For this review, take the finished solid that the model builds, in its own axes (mm). A direction names the side the tool comes from. Coordinates: 2 decimals unless noted, no trailing zeros. Loops run counter-clockwise (first coordinate to the right, second up) from the corner with the lowest first, then second, coordinate; pieces in that order, holes last. Notation, with made-up numbers: (60.25, -13) - (67.25, -13) arc R18 ccw to (67.25, 4) - close; hole circle Ø9 at (29.25, 1). An arc over 180 degrees is marked (long way). Answer as a JSON object with one key per item and string values. Group by question number.
Item 1: We need section A-A (y = 11.25). Give the boundary of the cut face in (x, z), then the cut area to 3 significant figures.
Item 2: We need section D-D (x = 21). Give the boundary of the cut face in (y, z).
Item 3: We need section C-C (y = 24.5). Give the boundary of the cut face in (x, z), then the cut area to 3 significant figures.
Item 4: Mouldability with a two-part tool opening along Y and no side actions: class faces 4 (the flat face through (56, 26.416, -18)), 5 (the cylindrical face through (57.34, 10.39, -18.41)), 6 (the cylindrical face through (4.996, 19.056, -18.406)), 7 (the flat face through (10.287, 16, -18)) as released by +Y, released by -Y, zero draft, split by the parting line, or undercut.
Item 5: Clearance check with flat-ended pins moving along their axes: pin 1 (4 mm diameter, centred on x = 55.26, y = 21.25, fed in from +Z); pin 2 (3 mm diameter, centred on x = 54.5, z = -3.5, fed in from +Y); pin 3 (1 mm diameter, centred on x = 37.5, z = -18.5, fed in from +Y); pin 4 (3 mm diameter, centred on x = 8, y = 14, fed in from +Z). State where each tip first meets the part, or that it passes through.
Item 6: To check wall thickness, follow line 1 (X direction, y = 0.9, z = -7.62); line 2 (Y direction, x = 18, z = -8.5); line 3 (X direction, y = 12.25, z = -18). State the ranges of each line that lie inside material, in increasing order.
Item 7: We need section B-B (z = -7.62). Give the boundary of the cut face in (x, y).
Item 8: Tool access review of faces 1 (the flat face through (60.96, 9, -18)), 2 (the flat face through (30, 1.27, -8)), 3 (the flat face through (30, 6.35, -18)): name each direction out of +Z, -Z, +X, -X, +Y, -Y from which nothing blocks a thin tool from reaching the whole face with its end or side.
from build123d import *

# Parameters (mm, degrees)
BOSS_EXTRUDE1_DEPTH    = 60.96
CONVERT_SOLID1_DEPTH   = 60.96
CONVERT_SOLID1_2_DEPTH = 60.96
SKETCH6_W              = 40.386
SKETCH6_H              = 20.066
CUT_EXTRUDE1_DEPTH     = 71.995158286
SKETCH8_R              = 1.89865
CUT_EXTRUDE2_DEPTH     = 71.767609116
SKETCH9_R              = 2.2479
CUT_EXTRUDE3_DEPTH     = 71.995158286
CUT_EXTRUDE4_DEPTH     = 71.995158286


# Read off the part's stored shape, not the designer's step: Convert-Solid1
with BuildPart() as part:
    # Sketch1 → Boss-Extrude1 (new body)
    with BuildSketch(Plane(origin=(0, 0, 0), x_dir=(0, 0, -1), z_dir=(1, 0, 0))):
        Polygon((0, 0), (19.05, 0), (19.05, 31.75), (17.78, 31.75), (17.78, 1.27), (0, 1.27), align=None)
    extrude(amount=BOSS_EXTRUDE1_DEPTH)

    # Convert-Solid1 outline → Convert-Solid1 (cut)
    with BuildSketch(Plane.YZ):
        with BuildLine():
            ThreePointArc((2.54, -19.05), (0.743948776, -18.306051224), (0, -16.51))
            Line((0, -16.51), (0, -19.05))
            Line((0, -19.05), (2.54, -19.05))
        make_face()
    extrude(amount=CONVERT_SOLID1_DEPTH, mode=Mode.SUBTRACT)

    # Convert-Solid1 2 outline → Convert-Solid1 2 (add)
    with BuildSketch(Plane.YZ):
        with BuildLine():
            ThreePointArc((2.54, -17.78), (1.641974388, -17.408025612), (1.27, -16.51))
            Line((1.27, -16.51), (1.27, -17.78))
            Line((1.27, -17.78), (2.54, -17.78))
        make_face()
    extrude(amount=CONVERT_SOLID1_2_DEPTH)

    # Sketch6 → Cut-Extrude1 (cut, through all)
    with BuildSketch(Plane.XY.offset(-17.78)):
        with Locations((30.48, 16.383)):
            Rectangle(SKETCH6_W, SKETCH6_H)
    extrude(amount=-CUT_EXTRUDE1_DEPTH, mode=Mode.SUBTRACT)

    # Sketch8 → Cut-Extrude2 (cut, through all)
    with BuildSketch(Plane(origin=(0, 1.27, 0), x_dir=(1, 0, 0), z_dir=(0, 1, 0))):
        with Locations(Location((7.62, 7.62, 0), (0, 0, 270))):
            Circle(SKETCH8_R)
        with Locations(Location((53.34, 7.62, 0), (0, 0, 270))):
            Circle(SKETCH8_R)
    extrude(amount=-CUT_EXTRUDE2_DEPTH, mode=Mode.SUBTRACT)

    # Sketch9 → Cut-Extrude3 (cut, through all)
    with BuildSketch(Plane.XY.offset(-17.78)):
        with Locations((5.483386699, 21.25)):
            Circle(SKETCH9_R)
        with Locations((5.483386699, 11.25)):
            Circle(SKETCH9_R)
        with Locations((55.262613301, 21.25)):
            Circle(SKETCH9_R)
        with Locations((55.262613301, 11.25)):
            Circle(SKETCH9_R)
    extrude(amount=-CUT_EXTRUDE3_DEPTH, mode=Mode.SUBTRACT)

    # Sketch10 → Cut-Extrude4 (cut, through all)
    with BuildSketch(Plane.XY.offset(-17.78)):
        Polygon((0, 26.416), (60.96, 26.416), (69.305073622, 29.055582779), (66.812292009, 41.145573602), (-9.342186268, 39.525265553), (-7.97115638, 29.055582779), (-7.223321897, 29.055582779), align=None)
    extrude(amount=-CUT_EXTRUDE4_DEPTH, mode=Mode.SUBTRACT)


solid = part.part
Check sheet entries:
{
 "1": {"outline": "(0, -19.05) - (3.24, -19.05) - (3.24, -17.78) - (0, -17.78) - close; (7.73, -19.05) - (10.29, -19.05) - (10.29, -17.78) - (7.73, -17.78) - close; (50.67, -19.05) - (53.01, -19.05) - (53.01, -17.78) - (50.67, -17.78) - close; (57.51, -19.05) - (60.96, -19.05) - (60.96, -17.78) - (57.51, -17.78) - close", "area": "14.7 mm2"},
 "2": {"outline": "(0, -16.51) arc R2.54 ccw to (2.54, -19.05) - (6.35, -19.05) - (6.35, -17.78) - (2.54, -17.78) arc R1.27 cw to (1.27, -16.51) - (1.27, 0) - (0, 0) - close"},
 "3": {"outline": "(0, -19.05) - (10.29, -19.05) - (10.29, -17.78) - (0, -17.78) - close; (50.67, -19.05) - (60.96, -19.05) - (60.96, -17.78) - (50.67, -17.78) - close", "area": "26.1 mm2"},
 "4": {"face 4": "released by +Y", "face 5": "undercut", "face 6": "undercut", "face 7": "zero draft"},
 "5": {"pin 1": "passes through", "pin 2": "stops at y = 1.27", "pin 3": "stops at y = 6.35", "pin 4": "stops at z = -17.78"},
 "6": {"line 1": "x = 0 to 5.72, 9.52 to 51.44, 55.24 to 60.96", "line 2": "y = 0 to 1.27", "line 3": "x = 0 to 3.47, 7.5 to 10.29, 50.67 to 53.25, 57.28 to 60.96"},
 "7": {"outline": "(0, 0) - (5.72, 0) - (5.72, 1.27) - (0, 1.27) - close; (9.52, 0) - (51.44, 0) - (51.44, 1.27) - (9.52, 1.27) - close; (55.24, 0) - (60.96, 0) - (60.96, 1.27) - (55.24, 1.27) - close"},
 "8": {"face 1": "+Z, -Z, +X, +Y, -Y", "face 2": "+Z, +X, -X, +Y", "face 3": "+Z, -Z, +Y"}
}
